The listing builds one solid part. Answer for the finished solid, in the listing's coordinates (mm). Round coordinates to 2 decimals unless told otherwise and drop trailing zeros. Write each loop counter-clockwise with the first axis right and the second up, starting at its lowest first coordinate (ties: lowest second). Pieces come first, ordered by that corner, then holes. Notation, with made-up numbers: M 8.25,32 L 20.25,32 A24 ccw 20.25,65 Z; hole C 18.5,31.25 d8. An arc over 180 degrees is marked long. Write each question's results on one line, items separated by ' | '.
Autodesk Inventor part; units mm, degrees
ref_plane "YZ Plane" through (0, 0, 0) normal (1, 0, 0) x (0, 1, 0)
ref_plane "XZ Plane" through (0, 0, 0) normal (0, 1, 0) x (-1, 0, 0)
ref_plane "XY Plane" through (0, 0, 0) normal (0, 0, 1) x (1, 0, 0)
sketch "スケッチ1" plane through (0, 0, 0) normal (0, 0, 1) x (1, 0, 0)
  circle A0 centre (0, 0) radius 11
  dimension "d0" = 22
extrude "押し出し1" add sketch "スケッチ1" along normal blind 2.16
sketch "スケッチ2" plane through (0, 0, 2.16) normal (0, 0, 1) x (1, 0, 0)
  circle A0 centre (0, 0) radius 5
  dimension "d3" = 10
extrude "押し出し2" add sketch "スケッチ2" along normal blind 10
sketch "スケッチ3" plane through (0, 0, 12.16) normal (0, 0, 1) x (1, 0, 0)
  circle A0 centre (0, 0) radius 1.565
  dimension "d6" = 3.13
extrude "押し出し3" cut sketch "スケッチ3" against normal up to surface (12.16 mm away)
sketch "スケッチ4" plane through (0, 0, 2.16) normal (0, 0, 1) x (1, 0, 0)
  circle A0 centre (0, 7.85) radius 1.35
  line L0 (0, -15.7768) -> (0, 17.6611)
  point P0 (0, 0)
  point P1 (0, 6.5)
  dimension "d9" = 2.7
  dimension "d10" = 6.5
extrude "押し出し4" cut sketch "スケッチ4" against normal up to surface (2.16 mm away)
pattern_circular "円形状パターン1" count 4 over 360 about axis through (0, 0, -10) along (0, 0, 1) of "押し出し4"
properties part number "frange"
1) Find the intervals of material crossed by line 1 (Y direction, x = 0, z = 0.7) (3 decimals); line 2 (Y direction, x = -0.75, z = 0.5); line 3 (Y direction, x = 0, z = 8.5) (3 decimals), in increasing order.
Return value:
line 1: -11 to -9.2, -6.5 to -1.565, 1.565 to 6.5, 9.2 to 11 | line 2: -10.97 to -8.97, -6.73 to -1.37, 1.37 to 6.73, 8.97 to 10.97 | line 3: -5 to -1.565, 1.565 to 5
2) The mould has two halves that part along X. Classify faces 1 (the face through (2, -5, 2.16)), 2 (the face through (-1.08, 4.88, 7.09)), 3 (the face through (-1.242, -0.952, 6.165)): +X half, -X half, draft (parallel to the pull), parting line (faces both ways), or undercut.
Return value:
face 1: draft | face 2: parting line | face 3: undercut
3) Section A-A (y = 0) is taken. Determine the outline of the cut face in (x, z) (3 decimals).
Return value:
outline: M -11,0 L -9.2,0 L -9.2,2.16 L -11,2.16 Z; M -6.5,0 L -1.565,0 L -1.565,12.16 L -5,12.16 L -5,2.16 L -6.5,2.16 Z; M 1.565,0 L 6.5,0 L 6.5,2.16 L 5,2.16 L 5,12.16 L 1.565,12.16 Z; M 9.2,0 L 11,0 L 11,2.16 L 9.2,2.16 Z
4) Section C-C (x = 7.85) is taken. Determine the outline of the cut face in (y, z), then the cut area to 3 significant figures.
Return value:
outline: M -7.71,0 L -1.35,0 L -1.35,2.16 L -7.71,2.16 Z; M 1.35,0 L 7.71,0 L 7.71,2.16 L 1.35,2.16 Z | area: 27.5 mm²
5) Each of these flat-tipped pins is pushed along its axis until it touches: pin 1 (5 mm diameter, centred on x = 3, y = 8, fed in from +Z); pin 2 (4.5 mm diameter, centred on x = 0, y = 7.85, fed in from -Z); pin 3 (1.5 mm diameter, centred on x = 1, z = 2, fed in from -Y); pin 4 (2 mm diameter, centred on y = -0.5, z = 5, fed in from -X). Where does it stop, or does it pass through?
Return value:
pin 1: z = 2.16 | pin 2: z = 0 | pin 3: y = -11 | pin 4: x = -5
